Source: CAD feature listing. Evaluate the final solid. Frame: model axes, mm. Face numbers are marked on the shaded views. A direction names the side the tool comes from. Coordinates: 2 decimals unless noted, no trailing zeros. Order: outer loops, then holes, each group sorted by start corner. A loop starts at its lowest first (then second) coordinate and runs counter-clockwise, first axis right, second up.
```python
from build123d import *

# Parameters (mm, degrees)
F0_W     = 100
F0_H     = 100
F1_DEPTH = 100
F2_T     = -5
F4_D     = 5.5


with BuildPart() as f1:
    # F0 (on Top) → F1 (new body)
    with BuildSketch(Plane.XY):
        Rectangle(F0_W, F0_H)
    extrude(amount=F1_DEPTH)

    # F2
    f2_openings = [f1.faces().sort_by_distance(p)[0] for p in [
        (0, -50, 50),
    ]]
    offset(amount=F2_T, openings=f2_openings)

    # F4 (through all)
    with Locations(Plane.XY.offset(100)):
        with Locations((0, -10)):
            Hole(F4_D / 2)


solid = f1.part
```
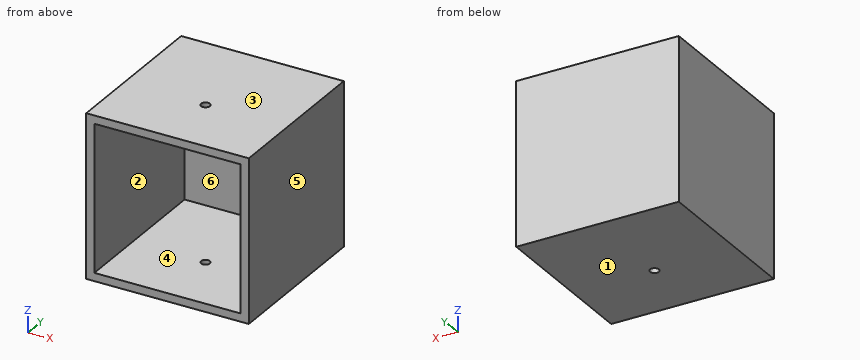
1. Section query D-D on y = -27.5. Return loops of the section in (x, z), plus the area to 3 significant figures.
Findings:
outline: (-50, 0) - (50, 0) - (50, 100) - (-50, 100) - close; hole (-45, 5) - (45, 5) - (45, 95) - (-45, 95) - close
area: 1,900 mm2
2. Section query C-C on z = 64. Return loops of the section in (x, y), plus the area to 3 significant figures.
Findings:
outline: (-50, -50) - (-45, -50) - (-45, 45) - (45, 45) - (45, -50) - (50, -50) - (50, 50) - (-50, 50) - close
area: 1,450 mm2
3. Draft query along X for the marked faces 3, 4, 5 and 6. Return one class per face: released by +X, released by -X, zero draft, split by the parting line, or undercut.
Findings:
face 3: zero draft
face 4: undercut
face 5: released by +X
face 6: undercut
4. Ray query, line 1 (Y direction, x = 0, z = 3.9); line 2 (X direction, y = 41.5, z = 44); line 3 (Z direction, x = 16, y = 22). Return the intervals inside material, ascending.
Findings:
line 1: y = -50 to -12.75, -7.25 to 50
line 2: x = -50 to -45, 45 to 50
line 3: z = 0 to 5, 95 to 100
5. Access query for the marked faces 1 and 2. Directions: +Z, -Z, +X, -X, +Y, -Y. A direction counts if a zero-diameter tool reaches every point of the face in a straight line with its end or side. Return the directions, or none.
Findings:
face 1: -Z, +X, -X, +Y, -Y
face 2: -Y
6. Section query A-A on y = -10. Return loops of the section in (x, z).
Findings:
outline: (-50, 0) - (-2.75, 0) - (-2.75, 5) - (-45, 5) - (-45, 95) - (-2.75, 95) - (-2.75, 100) - (-50, 100) - close; (2.75, 0) - (50, 0) - (50, 100) - (2.75, 100) - (2.75, 95) - (45, 95) - (45, 5) - (2.75, 5) - close
7. Pin query (flat end, axial travel): P1, Ø5, axis at x = 0, y = -10, coming from the -Z side; P2, Ø8, axis at x = -6, z = 82, coming from the -Y side. Return the tip coordinate at first contact, or that it passes through.
Findings:
P1: passes through
P2: stops at y = 45
8. Section query B-B on x = 0. Return loops of the section in (y, z).
Findings:
outline: (-50, 0) - (-12.75, 0) - (-12.75, 5) - (-50, 5) - close; (-50, 95) - (-12.75, 95) - (-12.75, 100) - (-50, 100) - close; (-7.25, 0) - (50, 0) - (50, 100) - (-7.25, 100) - (-7.25, 95) - (45, 95) - (45, 5) - (-7.25, 5) - close
